Model file for the job. Use its own axes, mm. A direction names the side the tool comes from. Coordinates: 2 decimals unless noted, no trailing zeros. Order: outer loops, then holes, each group sorted by start corner. A loop starts at its lowest first (then second) coordinate and runs counter-clockwise, first axis right, second up. Notation, with made-up numbers: M 27,79 L 53,79 A4 cw 53,86 Z; hole C -13.5,-38.75 d1. An arc over 180 degrees is marked long. Return JSON: item names as keys, results as strings.
```python
from build123d import *

# Parameters (mm, degrees)
SKETCH_1_W          = 40
SKETCH_1_H          = 40
SKETCH_1_R          = 2
SKETCH_1_R_2        = 12
EXTRUDE_1_DEPTH     = 3
SKETCH_2_W          = 35
SKETCH_2_H          = 40
EXTRUDE_2_DEPTH     = 3
SKETCH_3_W          = 3
SKETCH_3_H          = 40
EXTRUDE_3_DEPTH     = 40
EXTRUDE_4_DEPTH     = 2
EXTRUDE_5_DEPTH     = 2
SKETCH_6_R          = 1.5
SKETCH_6_W          = 28
SKETCH_6_H          = 24
CUT_EXTRUDE_1_DEPTH = 12
FILLET_1_R          = 3
SKETCH_7_W          = 28
SKETCH_7_H          = 28
CUT_EXTRUDE_2_DEPTH = 12
FILLET_2_R          = 3
CUT_EXTRUDE_3_DEPTH = 49
FILLET_3_R          = 3
FILLET_4_R          = 3
CUT_EXTRUDE_4_DEPTH = 10
FILLET_5_R          = 3


with BuildPart() as part:
    # 草图1 → 凸台-拉伸1 (new body)
    with BuildSketch(Plane.XY):
        Rectangle(SKETCH_1_W, SKETCH_1_H)
        with Locations((11.313708499, 11.313708499)):
            Circle(SKETCH_1_R, mode=Mode.SUBTRACT)
        with Locations((11.313708499, -11.313708499)):
            Circle(SKETCH_1_R, mode=Mode.SUBTRACT)
        with Locations((-11.313708499, -11.313708499)):
            Circle(SKETCH_1_R, mode=Mode.SUBTRACT)
        with Locations((-11.313708499, 11.313708499)):
            Circle(SKETCH_1_R, mode=Mode.SUBTRACT)
        Circle(SKETCH_1_R_2, mode=Mode.SUBTRACT)
    extrude(amount=EXTRUDE_1_DEPTH)

    # 草图2 → 凸台-拉伸2 (add)
    with BuildSketch(Plane.XY.offset(3)):
        with Locations((-37.5, 0)):
            Rectangle(SKETCH_2_W, SKETCH_2_H)
    extrude(amount=-EXTRUDE_2_DEPTH)

    # 草图3 → 凸台-拉伸3 (add)
    with BuildSketch(Plane.XY.offset(3)):
        with Locations((-53.5, 0)):
            Rectangle(SKETCH_3_W, SKETCH_3_H)
    extrude(amount=EXTRUDE_3_DEPTH)

    # 草图4 → 凸台-拉伸4 (add)
    with BuildSketch(Plane(origin=(0, 20, 0), x_dir=(1, 0, 0), z_dir=(0, 1, 0))):
        Polygon((-52, -43), (20, -3), (-52, -3), align=None)
    extrude(amount=-EXTRUDE_4_DEPTH)

    # 草图5 → 凸台-拉伸5 (add)
    with BuildSketch(Plane.XZ.offset(20)):
        Polygon((-52, 43), (-52, 3), (20, 3), align=None)
    extrude(amount=-EXTRUDE_5_DEPTH)

    # 草图6 → 切除-拉伸1 (cut)
    with BuildSketch(Plane(origin=(-52, 0, 0), x_dir=(0, 0, -1), z_dir=(1, 0, 0))):
        with Locations((-39, 14)):
            Circle(SKETCH_6_R)
        with Locations((-7, 14)):
            Circle(SKETCH_6_R)
        with Locations((-7, -14)):
            Circle(SKETCH_6_R)
        with Locations((-39, -14)):
            Circle(SKETCH_6_R)
        with Locations((-23, 0)):
            Rectangle(SKETCH_6_W, SKETCH_6_H)
    extrude(amount=-CUT_EXTRUDE_1_DEPTH, mode=Mode.SUBTRACT)

    # 圆角1
    fillet_1_edges = [part.edges().sort_by_distance(p)[0] for p in [
        (-53.5, -12, 37),
        (-53.5, 12, 37),
        (-53.5, 12, 9),
        (-53.5, -12, 9),
    ]]
    fillet(fillet_1_edges, radius=FILLET_1_R)

    # 草图7 → 切除-拉伸2 (cut)
    with BuildSketch(Plane.XY.offset(3)):
        with Locations((-34, 0)):
            Rectangle(SKETCH_7_W, SKETCH_7_H)
    extrude(amount=-CUT_EXTRUDE_2_DEPTH, mode=Mode.SUBTRACT)

    # 圆角2
    fillet_2_edges = [part.edges().sort_by_distance(p)[0] for p in [
        (-20, 14, 1.5),
        (-20, -14, 1.5),
        (-48, -14, 1.5),
        (-48, 14, 1.5),
    ]]
    fillet(fillet_2_edges, radius=FILLET_2_R)

    # 草图8 → 切除-拉伸3 (cut)
    with BuildSketch(Plane(origin=(0, 20, 0), x_dir=(1, 0, 0), z_dir=(0, 1, 0))):
        Polygon((-47, -34.502427699), (-47, -8), (0.704369859, -8), align=None)
    extrude(amount=-CUT_EXTRUDE_3_DEPTH, mode=Mode.SUBTRACT)

    # 圆角3
    fillet_3_edges = [part.edges().sort_by_distance(p)[0] for p in [
        (0.704369859, 19, 8),
        (-47, 19, 34.502427699),
        (-47, 19, 8),
    ]]
    fillet(fillet_3_edges, radius=FILLET_3_R)

    # 圆角4
    fillet_4_edges = [part.edges().sort_by_distance(p)[0] for p in [
        (0.704369859, -19, 8),
        (-47, -19, 34.502427699),
        (-47, -19, 8),
    ]]
    fillet(fillet_4_edges, radius=FILLET_4_R)

    # 草图9 → 切除-拉伸4 (cut)
    with BuildSketch(Plane.XY.offset(3)):
        with BuildLine():
            Line((-4.949747468, 12.02081528), (-1.998451999, 9.069519811))
            Line((-1.998451999, 9.069519811), (12.02081528, -4.949747468))
            Line((12.02081528, -4.949747468), (16.263455967, -9.192388155))
            ThreePointArc((16.263455967, -9.192388155), (17.142135624, -11.313708499), (16.263455967, -13.435028843))
            Line((16.263455967, -13.435028843), (13.435028843, -16.263455967))
            ThreePointArc((13.435028843, -16.263455967), (11.313708499, -17.142135624), (9.192388155, -16.263455967))
            Line((9.192388155, -16.263455967), (4.949747468, -12.02081528))
            Line((4.949747468, -12.02081528), (-9.069519811, 1.998451999))
            Line((-9.069519811, 1.998451999), (-12.02081528, 4.949747468))
            Line((-12.02081528, 4.949747468), (-16.263455967, 9.192388155))
            ThreePointArc((-16.263455967, 9.192388155), (-17.142135624, 11.313708499), (-16.263455967, 13.435028843))
            Line((-16.263455967, 13.435028843), (-13.435028843, 16.263455967))
            ThreePointArc((-13.435028843, 16.263455967), (-11.313708499, 17.142135624), (-9.192388155, 16.263455967))
            Line((-9.192388155, 16.263455967), (-4.949747468, 12.02081528))
        make_face()
    extrude(amount=-CUT_EXTRUDE_4_DEPTH, mode=Mode.SUBTRACT)

    # 圆角5
    fillet_5_edges = [part.edges().sort_by_distance(p)[0] for p in [
        (4.178090404, -11.249158216, 1.5),
        (-11.249158216, 4.178090404, 1.5),
        (-4.178090404, 11.249158216, 1.5),
        (11.249158216, -4.178090404, 1.5),
    ]]
    fillet(fillet_5_edges, radius=FILLET_5_R)


solid = part.part
```
Item 1: Saw through at C-C (x = -1). Write the cut outline in (y, z).
Check result:
{"outline": "M -20,0 L -11.96,0 L -11.96,3 L -18,3 L -18,14.67 L -20,14.67 Z; M 11.96,0 L 20,0 L 20,14.67 L 18,14.67 L 18,3 L 11.96,3 Z"}
Item 2: Saw through at A-A (z = 39). Write the cut outline in (x, y).
Check result:
{"outline": "M -55,-20 L -44.8,-20 L -44.8,-18 L -52,-18 L -52,-15.5 L -55,-15.5 Z; M -55,-12.5 L -52,-12.5 L -52,12.5 L -55,12.5 Z; M -55,15.5 L -52,15.5 L -52,18 L -44.8,18 L -44.8,20 L -55,20 Z"}
Item 3: Pull direction Z, two halves, no side cores. Call faces 1 (the cylindrical face through (17.14, -11.28, 1.52)), 2 (the cylindrical face through (-53.52, 11.14, 36.1)), 3 (the flat face through (-54, 0, 43)): +Z half, -Z half, draft (parallel to the pull), parting line (faces both ways), or undercut.
Check result:
{"face 1": "draft", "face 2": "undercut", "face 3": "+Z half"}
Item 4: Wall check: line 1 (Y direction, x = -53, z = 39); line 2 (Y direction, x = -1.5, z = 12); line 3 (X direction, y = -3, z = 6.5). Give the ranges that are in metal, low to high.
Check result:
{"line 1": "y = -20 to -15.5, -12.5 to 12.5, 15.5 to 20", "line 2": "y = -20 to -18, 18 to 20", "line 3": "x = -55 to -52"}
Item 5: Saw through at B-B (y = -7). Write the cut outline in (x, z).
Check result:
{"outline": "M -55,0 L -48,0 L -48,3 L -52,3 L -52,9 L -55,9 Z; M -55,37 L -52,37 L -52,43 L -55,43 Z; M -20,0 L -9.75,0 L -9.75,3 L -20,3 Z; M 14.07,0 L 20,0 L 20,3 L 14.07,3 Z"}
Item 6: 3-axis set-ups, long thin cutter, end or side, ignore diameter. For faces 4 (the cylindrical face through (-53.52, -11.14, 36.1)), 5 (the cylindrical face through (-20.86, 13.1, 1.48)), 6 (the flat face through (-17, 0, 3)), 7 (the flat face through (-47, 19, 20)): which of +Z, -Z, +X, -X, +Y, -Y reach the whole face in a straight line?
Check result:
{"face 4": "+X, -X", "face 5": "+Z, -Z", "face 6": "+Z, +X", "face 7": "+Y, -Y"}
Item 7: Saw through at D-D (z = 7). Write the cut outline in (x, y), and give its area (3 significant figures).
Check result:
{"outline": "M -55,-20 L 12.8,-20 L 12.8,-18 L -52,-18 L -52,-15.5 L -55,-15.5 Z; M -55,-12.5 L -52,-12.5 L -52,12.5 L -55,12.5 Z; M -55,15.5 L -52,15.5 L -52,18 L 12.8,18 L 12.8,20 L -55,20 Z", "area": "361 mm2"}
Item 8: Drop flat-ended pins along their axis: pin 1 Ø12 at (x, z) = (-27, 13.5) entering from +Y; pin 2 Ø2 at (y, z) = (-19, 21.5) entering from +X; pin 3 Ø2 at (x, y) = (-29.5, 19.5) entering from +Z; pin 4 Ø1.6 at (x, y) = (-24.5, -18.5) entering from +Z. Give the stop position or say it passes through.
Check result:
{"pin 1": "stops at y = 20", "pin 2": "stops at x = -11.5", "pin 3": "stops at z = 31.06", "pin 4": "stops at z = 28.17"}
